The listing builds one solid part. Answer for the finished solid, in the listing's coordinates (mm). Face numbers are marked on the shaded views. A direction names the side the tool comes from. Give positions to 0.01 mm unless a question says otherwise; leave off trailing zeros. Loops run counter-clockwise (first coordinate to the right, second up) from the corner with the lowest first, then second, coordinate; pieces in that order, holes last.
Item 1: Consider line 1 along Y through (x, z) = (-3, 16.75); line 2 along Z through (x, y) = (-7.25, -8); line 3 along Z through (x, y) = (10.25, 7.5). Determine where each line is inside the solid, lowest interval first.
Item 2: A tool of negligible diameter and unlimited length cuts with its end or side. For the marked faces 1 and 2, from which of +Z, -Z, +X, -X, +Y, -Y can it reach the whole face along a straight path? Write none if from no direction.
Item 3: Section A-A, the plane y = 0 is taken. Give the vertices of the cut face in (x, z), and give its area (3 significant figures).
Item 4: Section C-C, the plane z = 9 is taken. Give the vertices of the cut face in (x, y), and give its area (3 significant figures).
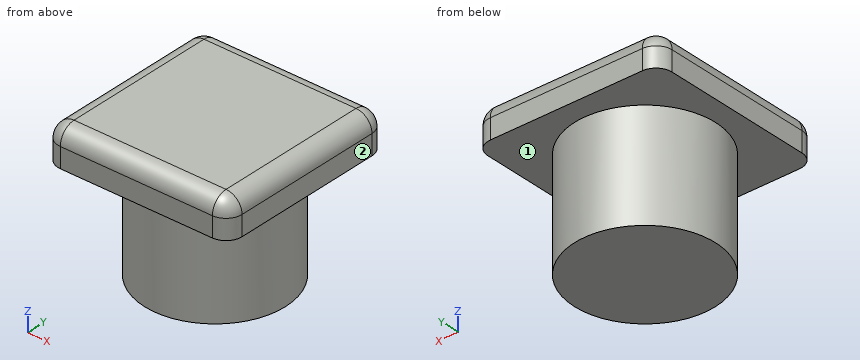
from build123d import *

# Parameters (mm, degrees)
SKETCH3_R           = 8.8
BOSS_EXTRUDE1_DEPTH = 13.5
SKETCH4_W           = 23
SKETCH4_H           = 23
BOSS_EXTRUDE2_DEPTH = 4.5
FILLET1_R           = 2


with BuildPart() as part:
    # Sketch3 → Boss-Extrude1 (new body)
    with BuildSketch(Plane.XY):
        Circle(SKETCH3_R)
    extrude(amount=BOSS_EXTRUDE1_DEPTH)

    # Sketch4 → Boss-Extrude2 (add)
    with BuildSketch(Plane.XY.offset(13.5)):
        Rectangle(SKETCH4_W, SKETCH4_H)
    extrude(amount=BOSS_EXTRUDE2_DEPTH)

    # Fillet1
    fillet1_edges = [part.edges().sort_by_distance(p)[0] for p in [
        (11.5, -11.5, 15.75),
        (11.5, 11.5, 15.75),
        (-11.5, 11.5, 15.75),
        (-11.5, -11.5, 15.75),
        (11.5, 0, 18),
        (0, 11.5, 18),
        (-11.5, 0, 18),
        (0, -11.5, 18),
    ]]
    fillet(fillet1_edges, radius=FILLET1_R)


solid = part.part
Worked answers:
1. line 1: y = -11.35 to 11.35
1. line 2: z = 13.5 to 18
1. line 3: z = 13.5 to 17.85
2. face 1: -Z
2. face 2: +Z, -Z, +X, +Y, -Y
3. outline: (-11.5, 13.5) - (-8.8, 13.5) - (-8.8, 0) - (8.8, 0) - (8.8, 13.5) - (11.5, 13.5) - (11.5, 16) arc R2 ccw to (9.5, 18) - (-9.5, 18) arc R2 ccw to (-11.5, 16) - close
3. area: 339 mm2
4. outline: circle Ø17.6 at (0, 0)
4. area: 243 mm2
